Design review of the part built by this model. Coordinates are the model's own, in mm. A direction names the side the tool comes from. Coordinates: 2 decimals unless noted, no trailing zeros. Loops run counter-clockwise (first coordinate to the right, second up) from the corner with the lowest first, then second, coordinate; pieces in that order, holes last. Notation, with made-up numbers: (-0.75, 34.25) -> (8.25, 34.25) arc R7 ccw to (8.25, 42.25) -> close; hole circle Ø3 at (24.5, -7). An arc over 180 degrees is marked (long way). Use a Markdown table: item, result. Add a question column.
Q1. Clearance check with flat-ended pins moving along their axes: pin 1 Ø0.8 at (y, z) = (-13, 24) entering from +X; pin 2 Ø1.5 at (x, y) = (2, -21.5) entering from +Z; pin 3 Ø7.5 at (y, z) = (-7.5, 15) entering from +X. State where each tip first meets the part, or that it passes through.
Q2. Take a section at B-B on x = -2. Write out the cut boundary in (y, z).
Q3. Take a section at C-C on z = 12.25. Write out the cut boundary in (x, y), plus the area to 3 significant figures.
Q4. Draft analysis for pull direction Y (two halves, no side actions). For faces 6 (the face through (2, -23, 15)), 7 (the face through (-13, 0, 13)), 8 (the face through (-5, -13, 24)), 9 (the face through (-10, -25, 13)), state which applies: pulls with the +Y half, pulls with the -Y half, needs draft (parallel to the pull), parting line crosses it, or undercut.
Q5. For probe 1 along Y at (x, z) = (3.25, 11.5); probe 2 along X at (y, z) = (-10.5, 20.75), list the stretches that pass through material, from the lowest coordinate up.
Q6. For faces 1 (the face through (-3, -12, 22.5)), 2 (the face through (-13, -12, 25)), 3 (the face through (2, -23, 10)), 4 (the face through (-13, -12, 0)), 5 (the face through (2, -20, 13)), list the 3-axis set-ups (+Z, -Z, +X, -X, +Y, -Y) from which the entire face can be reached by the end or side of a thin tool; tool diameter is ignored.
Q7. Take a section at D-D on y = -10.75. Write out the cut boundary in (x, z), plus the area to 4 significant figures.
Q8. Take a section at A-A on y = -23. Write out the cut boundary in (x, z), plus the area to 3 significant figures.
from build123d import *

# Parameters (mm, degrees)
F0_W     = 25
F0_H     = 25
F1_DEPTH = 25
F2_W     = 5
F2_H     = 5
F4_DEPTH = 5
F3_W     = 5
F3_H     = 5
F5_DEPTH = 2.5


with BuildPart() as f1:
    # F0 (on Front) → F1 (new body)
    with BuildSketch(Plane.XZ):
        with Locations((-12.5, 12.5)):
            Rectangle(F0_W, F0_H)
    extrude(amount=F1_DEPTH)

    # F2 (on face) → F4 (join)
    with BuildSketch(Plane.XZ.offset(25)):
        with Locations((2.5, 12.5)):
            Rectangle(F2_W, F2_H)
    extrude(amount=-F4_DEPTH)

    # F3 (on face) → F5 (cut, symmetric)
    with BuildSketch(Plane.XY.offset(25)):
        with Locations((-2.5, -12.5)):
            Rectangle(F3_W, F3_H)
    extrude(amount=F5_DEPTH, both=True, mode=Mode.SUBTRACT)


solid = f1.part
Answer list:
| question | item | result |
|---|---|---|
| 1 | pin 1 | x = -5 |
| 1 | pin 2 | z = 15 |
| 1 | pin 3 | x = 0 |
| 2 | outline | (-25, 0) -> (0, 0) -> (0, 25) -> (-10, 25) -> (-10, 22.5) -> (-15, 22.5) -> (-15, 25) -> (-25, 25) -> close |
| 3 | outline | (-25, -25) -> (5, -25) -> (5, -20) -> (0, -20) -> (0, 0) -> (-25, 0) -> close |
| 3 | area | 650 mm² |
| 4 | face 6 | needs draft |
| 4 | face 7 | pulls with the +Y half |
| 4 | face 8 | undercut |
| 4 | face 9 | pulls with the -Y half |
| 5 | probe 1 | -25 to -20 |
| 5 | probe 2 | -25 to 0 |
| 6 | face 1 | +Z, +X |
| 6 | face 2 | +Z, +X, -X, +Y, -Y |
| 6 | face 3 | -Z, +X, +Y, -Y |
| 6 | face 4 | -Z, +X, -X, +Y, -Y |
| 6 | face 5 | +Z, -Z, +X, +Y |
| 7 | outline | (-25, 0) -> (0, 0) -> (0, 22.5) -> (-5, 22.5) -> (-5, 25) -> (-25, 25) -> close |
| 7 | area | 612.5 mm² |
| 8 | outline | (-25, 0) -> (0, 0) -> (0, 10) -> (5, 10) -> (5, 15) -> (0, 15) -> (0, 25) -> (-25, 25) -> close |
| 8 | area | 650 mm² |
